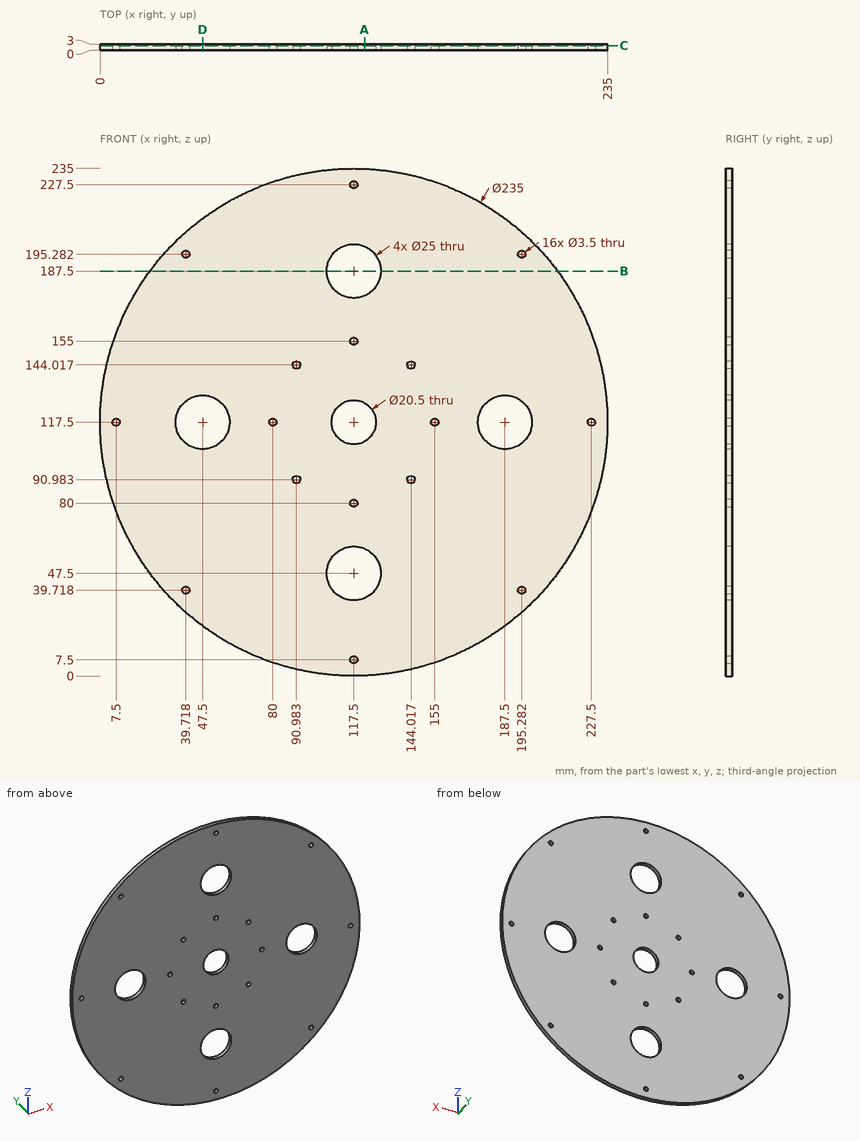
Design review of the part shown in the three views and the two pictorial views. Dimensions are in mm from the part's minimum x, y and z. Round coordinates to 2 decimals unless told otherwise and drop trailing zeros. Loops run counter-clockwise (first coordinate to the right, second up) from the corner with the lowest first, then second, coordinate; pieces in that order, holes last. Notation, with made-up numbers: (1.25, 9) -> (58.25, 9) arc R4 ccw to (58.25, 13) -> close; hole circle Ø8 at (28.5, -20.75). An arc over 180 degrees is marked (long way). Answer as CSV lines item,"result".
1) Add section A-A on x = 122.5. Write out the cut boundary in (y, z).
Geometry results:
outline,"(0, 0.11) -> (3, 0.11) -> (3, 36.04) -> (0, 36.04) -> close; (0, 58.96) -> (3, 58.96) -> (3, 108.55) -> (0, 108.55) -> close; (0, 126.45) -> (3, 126.45) -> (3, 176.04) -> (0, 176.04) -> close; (0, 198.96) -> (3, 198.96) -> (3, 234.89) -> (0, 234.89) -> close"
2) Add section D-D on x = 47.5. Write out the cut boundary in (y, z).
Geometry results:
outline,"(0, 23.13) -> (3, 23.13) -> (3, 105) -> (0, 105) -> close; (0, 130) -> (3, 130) -> (3, 211.87) -> (0, 211.87) -> close"
3) Add section B-B on z = 187.5. Write out the cut boundary in (x, y).
Geometry results:
outline,"(23.13, 0) -> (105, 0) -> (105, 3) -> (23.13, 3) -> close; (130, 0) -> (211.87, 0) -> (211.87, 3) -> (130, 3) -> close"
4) To check wall thickness, follow line 1 along X through (y, z) = (2.35, 41) (1 decimal); line 2 along X through (y, z) = (2.4, 91) (1 decimal); line 3 along X through (y, z) = (0.2, 185) (1 decimal). State the ranges of each line that lie inside material, in increasing order. Write a range as from..to.
Geometry results:
line 1,"x = 28.3..38.5, 40.9..106.8, 128.2..194.1, 196.5..206.7"
line 2,"x = 3..89.2, 92.7..142.3, 145.8..232"
line 3,"x = 21.3..105.3, 129.7..213.7"
5) Add section C-C on y = 2.25. State how many separate pieces and enclosed holes the cut face has, plus the area to 3 significant figures.
Geometry results:
separate pieces,"1"
enclosed holes,"21"
area,"40,900 mm²"
6) For P1, Ø1, axis at x = 142.5, z = 122.5, coming from the -Y side; P2, Ø3, axis at x = 39.72, z = 39.72, coming from the +Y side; P3, Ø1.5, axis at y = 1, z = 25.5, coming from the -X side (1 decimal), all flat-tipped, find the tip position at first contact; note any pin that passes through.
Geometry results:
P1,"stops at y = 0"
P2,"passes through"
P3,"stops at x = 43.5"
